Source: CAD feature listing. Evaluate the final solid. Frame: model axes, mm. A direction names the side the tool comes from. Coordinates: 2 decimals unless noted, no trailing zeros. Write each loop counter-clockwise with the first axis right and the second up, starting at its lowest first coordinate (ties: lowest second). Pieces come first, ordered by that corner, then holes. Notation, with made-up numbers: M 16.5,-12 L 59.5,-12 A7 cw 59.5,-1 Z; hole C -13,-12.75 d9. An arc over 180 degrees is marked long. Write item = value, one per line. Start each with the question number.
1. Access query for faces 5 (the face through (-28.884, 57, 13)), 6 (the face through (0, 57, 5.08)), 7 (the face through (32.52, 0.55, 23.87)), 8 (the face through (0, 57, 20.32)). Directions: +Z, -Z, +X, -X, +Y, -Y. A direction counts if a zero-diameter tool reaches every point of the face in a straight line with its end or side. Return the directions, or none.
2. Pull-direction query (X, two-part tool) for faces 1 (the face through (-26.343, 57, 12)), 2 (the face through (33.964, -1, 13)), 3 (the face through (-32.52, 42.5, 12.81)), 4 (the face through (0.404, -42.584, 1.528)); classes: pulls with the +X half, pulls with the -X half, needs draft (parallel to the pull), parting line crosses it, or undercut.
3. Pin query (flat end, axial travel): pin 1 Ø3 at (y, z) = (55, 10) entering from +X; pin 2 Ø12 at (x, z) = (2, 5) entering from +Y; pin 3 Ø8.5 at (y, z) = (52.5, 12) entering from -X; pin 4 Ø8.5 at (x, z) = (-2.5, 12) entering from +Y. Return the tip coordinate at first contact, or that it passes through.
4. Line query: line 1 along X through (y, z) = (52, 14.25); line 2 along Z through (x, y) = (19.5, 54.5); line 3 along Y through (x, z) = (-2, 15.5). Output: solid intervals per line, ascending.
5. Section query A-A (z = 13.25). Output: boundary loops of the cut face in (x, y).
6. Section query B-B (x = -24). Output: boundary loops of the cut face in (y, z), then the cut area to 3 significant figures.
```python
from build123d import *

# Parameters (mm, degrees)
F0_W     = 67.9279565811
F0_H     = 88.0647003651
F1_DEPTH = 25.4
F2_R     = 5.08
F3_DEPTH = 25.4
F4_W     = 52.0835686475
F4_H     = 10.6304162182
F5_DEPTH = 25.4


# Not quite as in the source:
# - a feature of the source that left no trace in its solid (it failed there, or was rolled back) is left out


with BuildPart() as f1:
    # F0 (on Top) → F1 (new body)
    with BuildSketch(Plane.XY):
        Rectangle(F0_W, F0_H)
    extrude(amount=F1_DEPTH)

    # F2
    f2_edges = [f1.edges().sort_by_distance(p)[0] for p in [
        (33.963978, -44.03235, 12.7),
        (33.963978, 44.03235, 12.7),
        (33.963978, 0, 0),
        (33.963978, 0, 25.4),
        (-33.963978, -44.03235, 12.7),
        (0, -44.03235, 0),
        (0, -44.03235, 25.4),
        (-33.963978, 44.03235, 12.7),
        (-33.963978, 0, 0),
        (-33.963978, 0, 25.4),
        (0, 44.03235, 0),
        (0, 44.03235, 25.4),
    ]]
    fillet(f2_edges, radius=F2_R)

    # F3 (add): a face of the model
    f3_faces = [f1.faces().sort_by_distance(p)[0] for p in [
        (0, 44.0323501825, 12.7),
    ]]
    extrude(f3_faces, amount=F3_DEPTH)

    # F4 (on face) → F5 (cut)
    with BuildSketch(Plane(origin=(0, 69.4323501825, 0), x_dir=(-1, 0, 0), z_dir=(0, 1, 0))):
        with Locations((0.3008237109, 12.2958261054)):
            Rectangle(F4_W, F4_H)
    extrude(amount=-F5_DEPTH, mode=Mode.SUBTRACT)


solid = f1.part
```
Results are:
q1.face_5 = +Z, -Z, -X, +Y
q1.face_6 = -Z, +X, -X, +Y
q1.face_7 = +Z, +X, +Y, -Y
q1.face_8 = +Z, +X, -X, +Y
q2.face_1 = undercut
q2.face_2 = pulls with the +X half
q2.face_3 = pulls with the -X half
q2.face_4 = needs draft
q3.pin_1 = 28.88
q3.pin_2 = 69.43
q3.pin_3 = -28.88
q3.pin_4 = 44.03
q4.line_1 = -28.88 to -26.34, 25.74 to 28.88
q4.line_2 = 5.08 to 6.98, 17.61 to 20.32
q4.line_3 = -44.03 to 44.03
q5.outline = M -33.96,-38.95 A5.08 ccw -28.88,-44.03 L 28.88,-44.03 A5.08 ccw 33.96,-38.95 L 33.96,38.95 A5.08 ccw 28.88,44.03 L 28.88,69.43 L 25.74,69.43 L 25.74,44.03 L -26.34,44.03 L -26.34,69.43 L -28.88,69.43 L -28.88,44.03 A5.08 ccw -33.96,38.95 Z
q6.outline = M -44.03,5.08 A5.08 ccw -38.95,0 L 38.95,0 A5.08 ccw 44.03,5.08 L 69.43,5.08 L 69.43,6.98 L 44.03,6.98 L 44.03,17.61 L 69.43,17.61 L 69.43,20.32 L 44.03,20.32 A5.08 ccw 38.95,25.4 L -38.95,25.4 A5.08 ccw -44.03,20.32 Z
q6.area = 2,330 mm^2
